Input: part model. Units: mm. Frame: model coordinates. Face numbers are marked on the shaded views. A direction names the side the tool comes from. Round coordinates to 2 decimals unless told otherwise and drop trailing zeros. Order: outer loops, then holes, each group sorted by start corner. A loop starts at its lowest first (then second) coordinate and runs counter-clockwise, first axis right, second up. Notation, with made-up numbers: (71.25, 7) -> (113.25, 7) arc R14 ccw to (113.25, 21) -> close; hole circle Ø3 at (-4.75, 41). An arc over 180 degrees is marked (long way). Use a Markdown table: item, result.
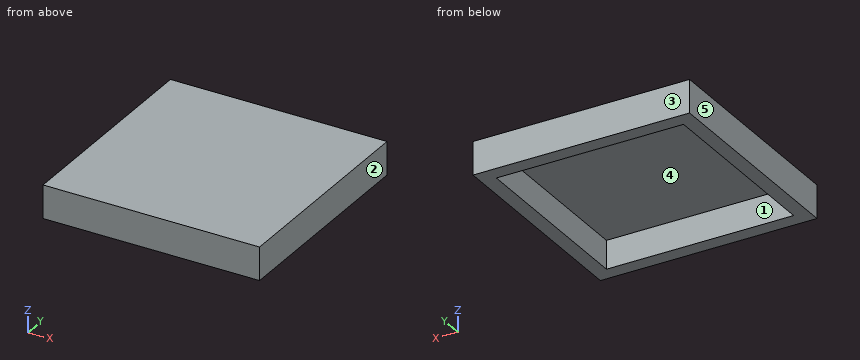
from build123d import *

# Parameters (mm, degrees)
SKETCH_1_W          = 70
SKETCH_1_H          = 70
EXTRUDE_1_DEPTH     = 10.7
SKETCH_2_W          = 60.5
SKETCH_2_H          = 60.5
CUT_EXTRUDE_1_DEPTH = 9.2


with BuildPart() as part:
    # Эскиз1 → Бобышка-Вытянуть1 (new body)
    with BuildSketch(Plane.XY):
        Rectangle(SKETCH_1_W, SKETCH_1_H)
    extrude(amount=-EXTRUDE_1_DEPTH)

    # Эскиз2 → Вырез-Вытянуть1 (cut)
    with BuildSketch(Plane(origin=(0, 0, -10.7), x_dir=(-1, 0, 0), z_dir=(0, 0, -1))):
        Rectangle(SKETCH_2_W, SKETCH_2_H)
    extrude(amount=-CUT_EXTRUDE_1_DEPTH, mode=Mode.SUBTRACT)


solid = part.part
1) Pin query (flat end, axial travel): pin 1 Ø5 at (x, y) = (-21.5, 0.5) entering from -Z. Return the tip coordinate at first contact, or that it passes through.
Results found:
| item | result |
|---|---|
| pin 1 | stops at z = -1.5 |
2) Cut plane A-A on z = -6. Return loops of the section in (x, y), and give its area (3 significant figures).
Results found:
| item | result |
|---|---|
| outline | (-35, -35) -> (35, -35) -> (35, 35) -> (-35, 35) -> close; hole (-30.25, -30.25) -> (30.25, -30.25) -> (30.25, 30.25) -> (-30.25, 30.25) -> close |
| area | 1,240 mm² |
3) Pull-direction query (X, two-part tool) for the marked faces 3, 4 and 5; classes: +X half, -X half, draft (parallel to the pull), parting line (faces both ways), or undercut.
Results found:
| item | result |
|---|---|
| face 3 | draft |
| face 4 | undercut |
| face 5 | -X half |
4) Cut plane B-B on x = -24. Return loops of the section in (y, z), and give its area (3 significant figures).
Results found:
| item | result |
|---|---|
| outline | (-35, -10.7) -> (-30.25, -10.7) -> (-30.25, -1.5) -> (30.25, -1.5) -> (30.25, -10.7) -> (35, -10.7) -> (35, 0) -> (-35, 0) -> close |
| area | 192 mm² |
5) Set-up query: the marked faces 1 and 2. Return all of +Z, -Z, +X, -X, +Y, -Y with unobstructed straight access to the full face (end or side cutting, diameter ignored); none if empty.
Results found:
| item | result |
|---|---|
| face 1 | -Z |
| face 2 | +Z, -Z, +X, +Y, -Y |
6) Line query: L1, parallel to X at y = 23, z = -6; L2, parallel to Z at x = 30, y = -5.5. Output: solid intervals per line, ascending. Write a range as [from, to].
Results found:
| item | result |
|---|---|
| L1 | x = [-35, -30.25], [30.25, 35] |
| L2 | z = [-1.5, 0] |
